Autodesk Inventor part; units mm, degrees
ref_plane "YZ Plane" through (0, 0, 0) normal (1, 0, 0) x (0, 1, 0)
ref_plane "XZ Plane" through (0, 0, 0) normal (0, 1, 0) x (-1, 0, 0)
ref_plane "XY Plane" through (0, 0, 0) normal (0, 0, 1) x (1, 0, 0)
sketch "Sketch1" plane through (0, 0, 0) normal (0, 0, 1) x (1, 0, 0)
  line L0 (-18.5, 0) -> (-18.5, 0.25)
  line L1 (-18.5, 0.25) -> (-13.5, 0.25)
  line L2 (-13.5, 0.25) -> (-13.5, 4.25)
  line L3 (-13.5, 4.25) -> (11.5, 4.25)
  line L4 (11.5, 4.25) -> (11.5, 3.75)
  line L5 (11.5, 3.75) -> (12, 3.75)
  line L6 (12, 3.75) -> (12, 4.25)
  line L7 (12, 4.25) -> (13.5, 4.25)
  line L8 (18.5, 0) -> (18.5, 0.25)
  line L9 (18.5, 0.25) -> (13.5, 4.25)
  line L10 (18.5, 0) -> (-18.5, 0)
  point P0 (0, 0)
  dimension "d0" = 0.25
  dimension "d1" = 5
  dimension "d2" = 4
  dimension "d8" = 25
  dimension "d9" = 0.5
  dimension "d10" = 0.5
  dimension "d11" = 0.5
  dimension "d12" = 1.5
  dimension "d14" = 0.25
revolve "Revolution1" add sketch "Sketch1" angle 360 about axis through (18.5, 0, 0) along (-1, 0, 0)
sketch "Sketch2" plane through (0, 0, 0) normal (0, 0, 1) x (1, 0, 0)
  line L0 (18.5, 0.25) -> (18.5, -0.25)
  line L1 (18.5, 0) -> (28.3, 0)
  line L2 (28.5, -0.2) -> (28.5, -10)
  arc A0 (28.5, -0.2) -> (28.3, 0) centre (28.3, -0.2) ccw
  point P0 (0, 0)
  point P1 (28.5, 0)
  dimension "d16" = 10
  dimension "d17" = 10
  dimension "d18" = 0.2
ref_plane "Work Plane1" through (18.5, 0, 0) normal (1, 0, 0) x (0, 0, -1)
sketch "Sketch3" plane through (18.5, 0, 0) normal (1, 0, 0) x (0, 0, -1)
  circle A0 centre (0, 0) radius 0.15
  dimension "d20" = 0.3
sweep "Sweep1" add profiles "Sketch3" path "Sketch2" path curves L1 A0 L2
mirror "Mirror1" about plane through (0, 0, 0) normal (1, 0, 0) of "Sweep1"
equation "\"BendRadius\" = Thickness"
equation "\"BendReliefWidth\" = Thickness"
equation "\"BendReliefDepth\" = 0.5 * Thickness"
equation "\"CornerReliefSize\" = 4 * Thickness"
equation "\"MinimumRemnant\" = 2 * Thickness"
equation "\"TransitionRadius\" = BendRadius"
equation "\"JacobiRadiusSize\" = BendRadius"
equation "\"GapSize\" = Thickness"
properties part number "K50-29"
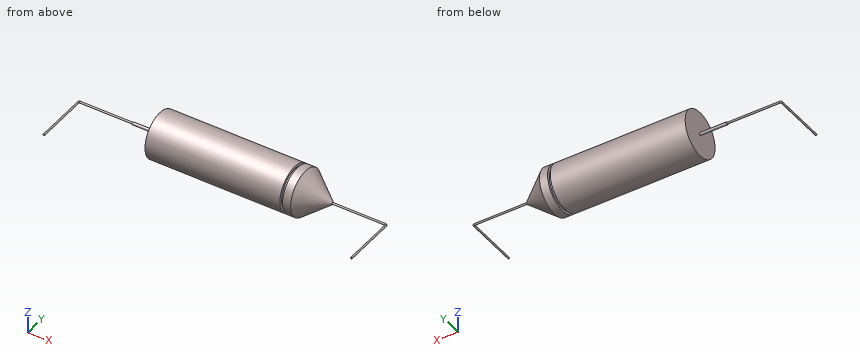
Part model, mm, in its own coordinate system. Round coordinates to 2 decimals unless told otherwise and drop trailing zeros. Order: outer loops, then holes, each group sorted by start corner. A loop starts at its lowest first (then second) coordinate and runs counter-clockwise, first axis right, second up. Notation, with made-up numbers: M 41,48 L 61,48 A27 cw 61,66 Z; hole C -3.5,-16 d10. An arc over 180 degrees is marked long. Answer in a Markdown table with one row per item. Add a question column.
Q1. Pin check, flat tips, straight feed: pin 1 (1 mm diameter, centred on y = -4, z = -1.5, fed in from -X); pin 2 (8 mm diameter, centred on x = -20, y = 0.5, fed in from +Z). Stop position of each tip, or through.
Q2. Cut at B-B on x = 16. Give the cut face in (y, z).
Q3. Wall check: L1, parallel to X at y = -2.75, z = 0 (3 decimals); L2, parallel to X at y = -1.75, z = 0 (3 decimals); L3, parallel to Y at x = 3.5, z = -0.25. Give the ranges that are in metal, low to high. Write a range as from..to.
Q4. Cut at A-A on y = -7. Give the cut face in (x, z).
Established:
| question | item | result |
|---|---|---|
| 1 | pin 1 | stops at x = -13.5 |
| 1 | pin 2 | stops at z = 0.25 |
| 2 | outline | C 0,0 d4.5 |
| 3 | L1 | x = -28.65..-28.35, -13.5..15.375, 28.35..28.65 |
| 3 | L2 | x = -28.65..-28.35, -13.5..16.625, 28.35..28.65 |
| 3 | L3 | y = -4.24..4.24 |
| 4 | outline | C -28.5,0 d0.3; C 28.5,0 d0.3 |
